Read the model definition and answer for the solid it produces. Units are mm, in the model's axes. A direction names the side the tool comes from. Coordinates: 2 decimals unless noted, no trailing zeros. Loops run counter-clockwise (first coordinate to the right, second up) from the corner with the lowest first, then second, coordinate; pieces in that order, holes last.
from build123d import *

# Parameters (mm, degrees)
SKIZZE1_W                        = 35
SKIZZE1_H                        = 75
AUFSATZ_LINEAR_AUSTRAGEN1_DEPTH  = 1.5
SKIZZE3_W                        = 15.25
SKIZZE3_H                        = 5
SKIZZE3_W_2                      = 4.875
SCHNITT_LINEAR_AUSTRAGEN12_DEPTH = 20
SKIZZE10_R                       = 12
SKIZZE10_R_2                     = 11
SCHNITT_LINEAR_AUSTRAGEN16_DEPTH = 1.5
SCHNITT_LINEAR_AUSTRAGEN17_DEPTH = 1.5
SKIZZE12_W                       = 1
SKIZZE12_H                       = 28.144103088
AUFSATZ_LINEAR_AUSTRAGEN7_DEPTH  = 1.5


with BuildPart() as part:
    # Skizze1 → Aufsatz-Linear austragen1 (new body)
    with BuildSketch(Plane.XY):
        with Locations((17.5, 37.5)):
            Rectangle(SKIZZE1_W, SKIZZE1_H)
    extrude(amount=AUFSATZ_LINEAR_AUSTRAGEN1_DEPTH)

    # Skizze3 → Schnitt-Linear austragen12 (cut)
    with BuildSketch(Plane.XY.offset(1.5)):
        with Locations((17.5, 2.5)):
            Rectangle(SKIZZE3_W, SKIZZE3_H)
        with Locations((32.5625, 2.5)):
            Rectangle(SKIZZE3_W_2, SKIZZE3_H)
        with Locations((2.4375, 2.5)):
            Rectangle(SKIZZE3_W_2, SKIZZE3_H)
    extrude(amount=-SCHNITT_LINEAR_AUSTRAGEN12_DEPTH, mode=Mode.SUBTRACT)

    # Skizze10 → Schnitt-Linear austragen16 (cut)
    with BuildSketch(Plane.XY.offset(1.5)):
        with Locations((17.5, 29)):
            Circle(SKIZZE10_R)
        with Locations((17.5, 29)):
            Circle(SKIZZE10_R_2, mode=Mode.SUBTRACT)
    extrude(amount=-SCHNITT_LINEAR_AUSTRAGEN16_DEPTH, mode=Mode.SUBTRACT)


with BuildPart() as schnitt_linear_austragen16_piece_1:
    # of the separate pieces the step leaves, piece 1, a body of its own (schnitt_linear_austragen16_pieces)
    add(part.part.solids().sort_by_distance((4.875, 0, 0))[0])


with BuildPart() as schnitt_linear_austragen16_piece_2:
    # of the separate pieces the step leaves, piece 2, a body of its own (schnitt_linear_austragen16_pieces)
    add(part.part.solids().sort_by_distance((28.5, 29, 0))[0])


with BuildPart() as schnitt_linear_austragen17_tool:
    # Skizze11 → Schnitt-Linear austragen17 (new body)
    with BuildSketch(Plane.XY.offset(1.5)):
        Polygon((28.268155747, 64.5), (29.5, 64.5), (8.288020016, 35.011607504), (7.787416934, 36.04739173), align=None)
    extrude(amount=-SCHNITT_LINEAR_AUSTRAGEN17_DEPTH)


with BuildPart() as schnitt_linear_austragen16_piece_1_1:
    add(schnitt_linear_austragen16_piece_1.part)

    # Schnitt-Linear austragen17: cut by schnitt_linear_austragen17_tool
    add(schnitt_linear_austragen17_tool.part, mode=Mode.SUBTRACT)



with BuildPart() as schnitt_linear_austragen16_piece_2_1:
    add(schnitt_linear_austragen16_piece_2.part)

    # Schnitt-Linear austragen17: cut by schnitt_linear_austragen17_tool
    add(schnitt_linear_austragen17_tool.part, mode=Mode.SUBTRACT)


with BuildPart() as schnitt_linear_austragen16_piece_1_2:
    add(schnitt_linear_austragen16_piece_1_1.part)

    add(schnitt_linear_austragen16_piece_2_1.part)  # Aufsatz-Linear austragen7 merges Schnitt-Linear austragen16 piece 2
    # Skizze12 → Aufsatz-Linear austragen7 (add)
    with BuildSketch(Plane.XY.offset(1.5)):
        with Locations((17.5, 28.571124528)):
            Rectangle(SKIZZE12_W, SKIZZE12_H)
    extrude(amount=-AUFSATZ_LINEAR_AUSTRAGEN7_DEPTH)


solid = schnitt_linear_austragen16_piece_1_2.part
Q1. Flat-ended cylindrical pins translate along their axes: pin 1 Ø0.8 at (y, z) = (3, 1) entering from -X (3 decimals); pin 2 Ø0.8 at (y, z) = (2, 0.5) entering from +X (3 decimals). Find the tip coordinate at first contact, or state that the pin passes through.
Findings below:
pin 1: stops at x = 4.875
pin 2: stops at x = 30.125
Q2. Which of the six approach directions +Z, -Z, +X, -X, +Y, -Y give full straight-line access (tool end or side, diameter ignored) to faces 1 (the face through (17, 38, 0)), 2 (the face through (17, 5, 1)), 3 (the face through (30.125, 2, 1)), 4 (the face through (4.875, 2, 1)), 5 (the face through (12.5, 38.8, 0.8))?
Findings below:
face 1: -Z, +X, -X, +Y, -Y
face 2: +Z, -Z, -Y
face 3: +Z, -Z, +X, -Y
face 4: +Z, -Z, -X, -Y
face 5: +Z, -Z
Q3. A cutting plane is placed at D-D (y = 52). Give the vertices of the cut face in (x, z), then the cut area to 3 significant figures.
Findings below:
outline: (0, 0) - (19.27, 0) - (19.27, 1.5) - (0, 1.5) - close; (20.51, 0) - (35, 0) - (35, 1.5) - (20.51, 1.5) - close
area: 50.6 mm2
Q4. A cutting plane is placed at A-A (z = 0.9). Give the vertices of the cut face in (x, y) (3 decimals), then the cut area to 3 significant figures.
Findings below:
outline: (0, 5) - (4.875, 5) - (4.875, 0) - (9.875, 0) - (9.875, 5) - (25.125, 5) - (25.125, 0) - (30.125, 0) - (30.125, 5) - (35, 5) - (35, 75) - (0, 75) - close; hole (7.787, 36.047) arc R12 ccw to (17, 17.01) - (17, 18.011) arc R11 cw to (8.288, 35.012) - (8.871, 35.822) arc R11 cw to (17, 39.989) - (17, 40.99) arc R12 ccw to (11.395, 39.331) - (29.5, 64.5) - (28.268, 64.5) - close; hole (18, 17.01) arc R12 ccw to (18, 40.99) - (18, 39.989) arc R11 cw to (18, 18.011) - close
area: 2,400 mm2
Q5. A cutting plane is placed at C-C (y = 29). Give the vertices of the cut face in (x, z), then the cut area to 3 significant figures.
Findings below:
outline: (0, 0) - (5.5, 0) - (5.5, 1.5) - (0, 1.5) - close; (6.5, 0) - (28.5, 0) - (28.5, 1.5) - (6.5, 1.5) - close; (29.5, 0) - (35, 0) - (35, 1.5) - (29.5, 1.5) - close
area: 49.5 mm2
Q6. Determine the mould class of faces 6 (the face through (28.5, 28.8, 0.8)), 7 (the face through (9.875, 2, 1)), 8 (the face through (0, 40, 1)), 9 (the face through (7, 0, 1)) for opening direction X: +X half, -X half, draft (parallel to the pull), parting line (faces both ways), or undercut.
Findings below:
face 6: undercut
face 7: undercut
face 8: -X half
face 9: draft
Q7. A cutting plane is placed at B-B (x = 26.5). Give the vertices of the cut face in (y, z).
Findings below:
outline: (0, 0) - (21.06, 0) - (21.06, 1.5) - (0, 1.5) - close; (22.68, 0) - (35.32, 0) - (35.32, 1.5) - (22.68, 1.5) - close; (36.94, 0) - (60.33, 0) - (60.33, 1.5) - (36.94, 1.5) - close; (62.04, 0) - (75, 0) - (75, 1.5) - (62.04, 1.5) - close
Q8. Straight lines are drawn through the part: probe 1 along X at (y, z) = (29.5, 0.8); probe 2 along Y at (x, z) = (10, 0.95); probe 3 along Y at (x, z) = (25, 0.3). For each, find the intervals that lie inside material, in ascending order.
Findings below:
probe 1: x = 0 to 5.51, 6.51 to 28.49, 29.49 to 35
probe 2: y = 5 to 19.63, 20.95 to 37.05, 39.12 to 75
probe 3: y = 5 to 19.63, 20.95 to 37.05, 38.37 to 58.24, 59.96 to 75
